The drawing under review shows one solid part. Ordinate dimensions are in mm from its lowest x, y, z. Give positions to 0.01 mm unless a question says otherwise; leave off trailing zeros. Write each loop counter-clockwise with the first axis right and the second up, starting at its lowest first coordinate (ties: lowest second). Pieces come first, ordered by that corner, then holes. Notation, with made-up numbers: M -7,60 L -1,60 A19 ccw -1,66 Z; hole C 76,-6 d2. An arc over 180 degrees is marked long. One line per item, written item: value. Start each with the question number.
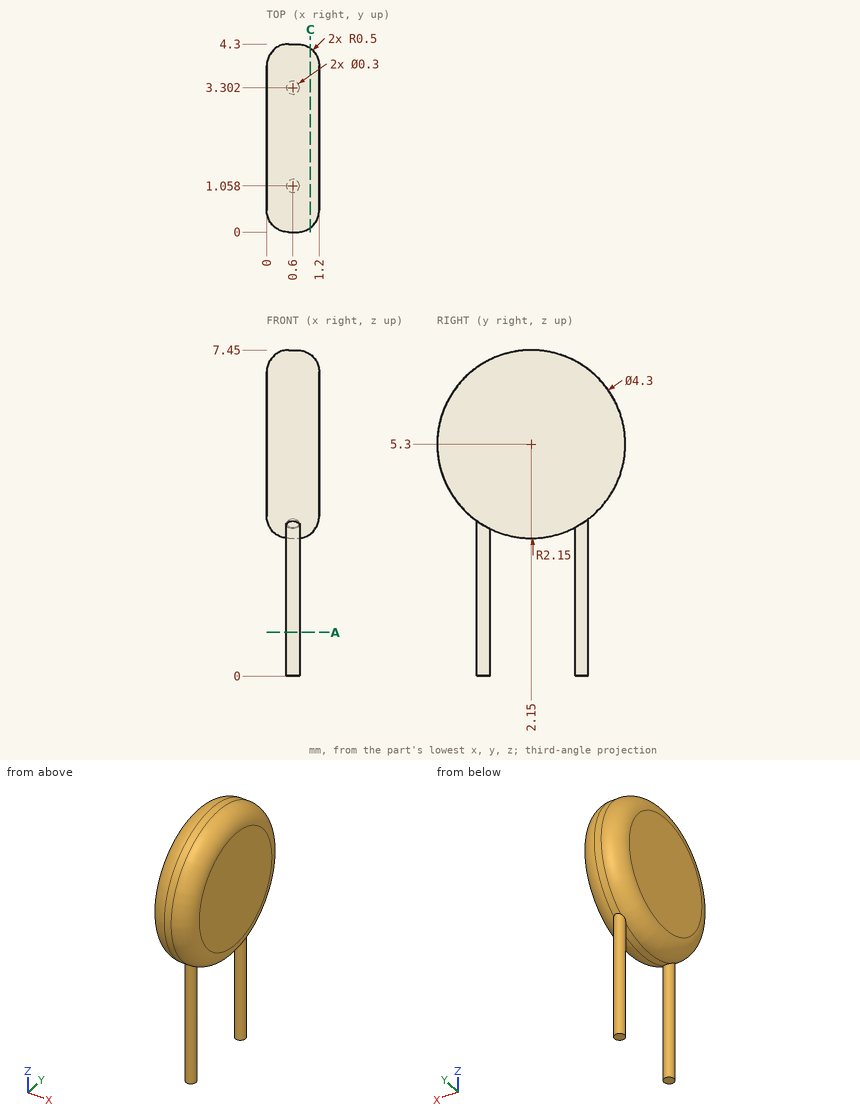
Q1. Take a section at A-A, the plane z = 1. Give the boundary of the cut face in (x, y).
Q2. Take a section at C-C, the plane x = 1. Give the boundary of the cut face in (y, z).
Q3. Wall thickness on line 1 (Z direction, x = 0.9, y = 3.4); line 2 (Y direction, x = 0.2, z = 4) (1 decimal); line 3 (Z direction, x = 0.15, y = 0.65) (1 decimal): over which ranges is each line inside the solid? List them lowest first. Write a range as from..to.
Results list:
1. outline: C 0.6,1.06 d0.3; C 0.6,3.3 d0.3
2. outline: C 2.15,5.3 d4.1
3. line 1: z = 3.6..7
3. line 2: y = 0.6..3.7
3. line 3: z = 4..6.6
